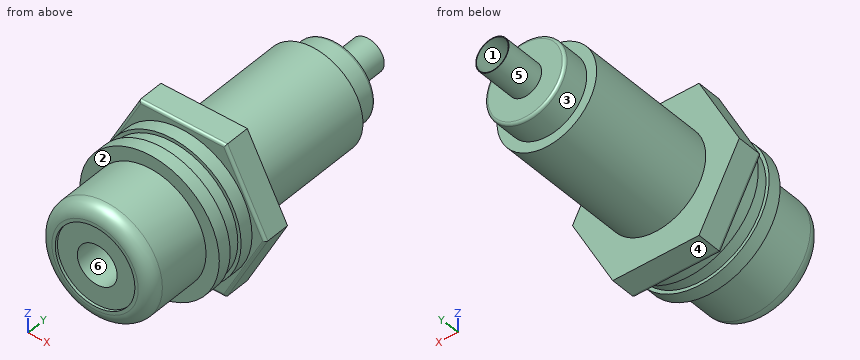
Solid Edge part; units mm, degrees
sketch "Sketch1" plane through (0, 0, 0) normal (0, -1, 0) x (1, 0, 0)
  line L0 (-3.25, 5.75) -> (3.25, 5.75)
  line L1 (3.25, 5.75) -> (6.2811, 0)
  line L2 (6.2811, 0) -> (3.25, -5.75)
  line L3 (3.25, -5.75) -> (-3.25, -5.75)
  line L4 (-3.25, -5.75) -> (-6.2811, 0)
  line L5 (-6.2811, 0) -> (-3.25, 5.75)
  dimension "D1" = 3.25
  dimension "D2" = 3.25
  dimension "D3" = 6.2811
  dimension "D4" = 6.2811
  dimension "D5" = 3.25
  dimension "D6" = 3.25
  dimension "D7" = 3.25
  dimension "D8" = 6.2811
extrude "Protrusion1" add sketch "Sketch1" against normal blind 2
fillet "Verrundung_1" radius 0.2 6 edges at (-4.7655, 0, 2.875) (0, 0, 5.75) (4.7655, 0, 2.875) (4.7655, 0, -2.875) (0, 0, -5.75) (-4.7655, 0, -2.875)
sketch "Sketch2" plane through (0, 0, 0) normal (0, -1, 0) x (1, 0, 0)
  circle A0 centre (0, 0) radius 5.25
extrude "Ausprägung_2" add sketch "Sketch2" along normal blind 1
sketch "Sketch3" plane through (0, -1, 0) normal (0, -1, 0) x (1, 0, 0)
  circle A0 centre (0, 0) radius 5
extrude "Ausprägung_3" add sketch "Sketch3" along normal blind 1
sketch "Sketch4" plane through (0, -2, 0) normal (0, -1, 0) x (1, 0, 0)
  circle A0 centre (0, 0) radius 5.25
extrude "Ausprägung_4" add sketch "Sketch4" along normal blind 1
sketch "Sketch5" plane through (0, -3, 0) normal (0, -1, 0) x (1, 0, 0)
  circle A0 centre (0, 0) radius 4.25
extrude "Ausprägung_5" add sketch "Sketch5" along normal blind 5
sketch "Sketch6" plane through (0, -8, 0) normal (0, -1, 0) x (1, 0, 0)
  circle A0 centre (0, 0) radius 3
extrude "Ausschnitt_2" cut sketch "Sketch6" against normal blind 0.2
sketch "Sketch7" plane through (0, 2, 0) normal (0, 1, 0) x (-1, 0, 0)
  circle A0 centre (0, 0) radius 3.75
extrude "Ausprägung_6" add sketch "Sketch7" along normal blind 10
sketch "Sketch8" plane through (0, 12, 0) normal (0, 1, 0) x (-1, 0, 0)
  circle A0 centre (0, 0) radius 3
extrude "Ausprägung_7" add sketch "Sketch8" along normal blind 2
sketch "Sketch9" plane through (0, 14, 0) normal (0, 1, 0) x (-1, 0, 0)
  circle A0 centre (0, 0) radius 1.25
extrude "Ausprägung_8" add sketch "Sketch9" along normal blind 3
sketch "Sketch10" plane through (0, 17, 0) normal (0, 1, 0) x (-1, 0, 0)
  circle A0 centre (0, 0) radius 1.2
extrude "Ausschnitt_3" cut sketch "Sketch10" against normal blind 2.8
sketch "Sketch11" plane through (0, -7.8, 0) normal (0, -1, 0) x (1, 0, 0)
  circle A0 centre (0, 0) radius 1.5
extrude "Ausschnitt_4" cut sketch "Sketch11" against normal blind 19
fillet "Verrundung_2" radius 1 1 edges at (-4.25, -8, 0)
fillet "Verrundung_3" radius 0.2 1 edges at (3, 14, 0)
Model file for the job. Use its own axes, mm. Face numbers are marked on the shaded views. A direction names the side the tool comes from. Coordinates: 2 decimals unless noted, no trailing zeros. Order: outer loops, then holes, each group sorted by start corner. A loop starts at its lowest first (then second) coordinate and runs counter-clockwise, first axis right, second up. Notation, with made-up numbers: (31, 75.25) -> (39, 75.25) arc R19 ccw to (39, 108.25) -> close; hole circle Ø11 at (-37.75, -15.5). An arc over 180 degrees is marked (long way). Return JSON: item names as keys, results as strings. Group by question number.
Item 1: Tool access for the marked faces 4, 5 and 6: list every direction of +Z, -Z, +X, -X, +Y, -Y with a clear straight run to the whole face (end or side of a thin tool).
Item 2: Pull direction Z, two halves, no side cores. Call the marked faces 1, 2 and 3: pulls with the +Z half, pulls with the -Z half, needs draft (parallel to the pull), parting line crosses it, or undercut.
Item 3: Flat gauge pins, fed straight in: P1, Ø1, axis at x = 4.5, z = -2, coming from the -Y side; P2, Ø2.5, axis at x = -0.5, z = 0.5, coming from the -Y side; P3, Ø6, axis at x = -2, z = -4, coming from the +Y side. Where does each tip first touch, or does it go through?
Item 4: Saw through at B-B on y = 14.75. Write the cut outline in (x, z).
Item 5: Saw through at C-C on y = 4. Write the cut outline in (x, z), then the cut area to 3 significant figures.
Item 6: Wall check: line 1 along Y through (x, z) = (-3, -4.25); line 2 along X through (y, z) = (11.5, 2.5); line 3 along Z through (x, y) = (-0.25, 7.75). Give the ranges that are in metal, low to high. Write a range as [from, to].
Item 7: Saw through at A-A on y = 1. Write the cut outline in (x, z), then the cut area to 3 significant figures.
Values found:
{
 "1": {"face 4": "-Z, +X, -X, +Y, -Y", "face 5": "+Y", "face 6": "-Y"},
 "2": {"face 1": "undercut", "face 2": "needs draft", "face 3": "parting line crosses it"},
 "3": {"P1": "stops at y = -3", "P2": "stops at y = -7.8", "P3": "stops at y = 14"},
 "4": {"outline": "circle Ø2.5 at (0, 0); hole circle Ø2.4 at (0, 0)"},
 "5": {"outline": "circle Ø7.5 at (0, 0); hole circle Ø3 at (0, 0)", "area": "37.1 mm2"},
 "6": {"line 1": "y = [-3, -2], [-1, 2]", "line 2": "x = [-2.8, 2.8]", "line 3": "z = [-3.74, -1.48], [1.48, 3.74]"},
 "7": {"outline": "(-6.28, 0) -> (-3.25, -5.75) -> (3.25, -5.75) -> (6.28, 0) -> (3.25, 5.75) -> (-3.25, 5.75) -> close; hole circle Ø3 at (0, 0)", "area": "103 mm2"}
}
